Build history of the part. All positions in model axes, mm. Face numbers are marked on the shaded views. Round coordinates to 2 decimals unless told otherwise and drop trailing zeros. Write each loop counter-clockwise with the first axis right and the second up, starting at its lowest first coordinate (ties: lowest second). Pieces come first, ordered by that corner, then holes. Notation, with made-up numbers: M 72.5,38.5 L 118.5,38.5 A25 ccw 118.5,76.5 Z; hole C -20.5,52 d9. An arc over 180 degrees is marked long. Write item = value, one per line. Start each with the question number.
Q1. Band-saw the part on A-A on x = 11.25. Write the cut outline in (y, z), plus the area to 3 significant figures.
Q2. Band-saw the part on C-C on z = -12. Write the cut outline in (x, y), plus the area to 3 significant figures.
Q3. Band-saw the part on B-B on y = 0.9. State how many separate pieces and enclosed holes the cut face has, plus the area to 3 significant figures.
Q4. Drop flat-ended pins along their axis: P1, Ø0.5, axis at x = 11.5, y = 1, coming from the +Z side; P2, Ø5, axis at x = 6.5, z = -112.5, coming from the +Y side; P3, Ø0.8, axis at y = 0.5, z = -6.5, coming from the -X side. Give the stop position or say it passes through.
Q5. Pull direction Z, two halves, no side cores. Call the marked faces 1 and 2: released by +Z, released by -Z, zero draft, split by the parting line, or undercut.
Q6. Probe L1, parallel to Z at x = 16.5, y = 1.1; L2, parallel to Z at x = 8.75, y = 0.7; L3, parallel to Z at x = 6.5, y = 0.6. List the from-to ranges inside material, lowest first.
Q7. Band-saw the part on D-D on z = -114.5. Write the cut outline in (x, y).
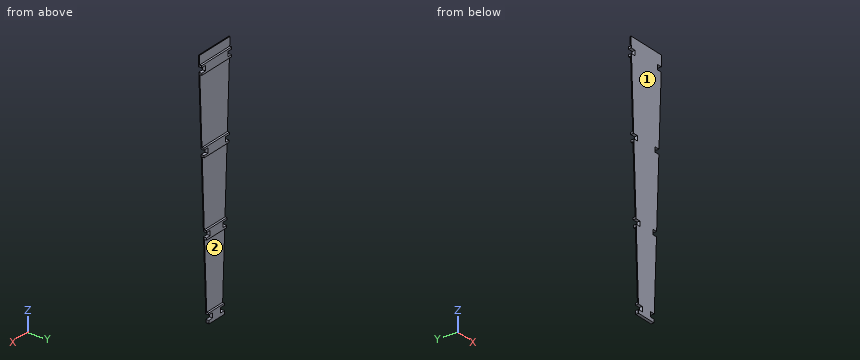
```python
from build123d import *

# Parameters (mm, degrees)
BOSS_EXTRUDE1_DEPTH = 0.5
BOSS_EXTRUDE2_DEPTH = 1


with BuildPart() as part:
    # Sketch2 → Boss-Extrude1 (new body)
    with BuildSketch(Plane(origin=(0, 0, 0), x_dir=(1, 0, 0), z_dir=(0, 1, 0))):
        Polygon((0.216060204, 5.401505112), (0, 0), (20, 0), (19.783939796, 5.401505112), (17.280808425, 5.401505112), (17.280808425, 7.904636482), (19.683814541, 7.904636482), (18.245170319, 43.870742022), (15.742038949, 43.870742022), (15.742038949, 46.373873393), (18.145045064, 46.373873393), (16.706400843, 82.339978933), (14.203269472, 82.339978933), (14.203269472, 84.843110303), (16.606275588, 84.843110303), (15.167631366, 120.809215844), (12.664499996, 120.809215844), (12.664499996, 123.312347214), (15.067506111, 123.312347214), (15, 125), (5, 125), (4.932493889, 123.312347214), (7.335500004, 123.312347214), (7.335500004, 120.809215844), (4.832368634, 120.809215844), (3.393724412, 84.843110303), (5.796730528, 84.843110303), (5.796730528, 82.339978933), (3.293599157, 82.339978933), (1.854954936, 46.373873393), (4.257961051, 46.373873393), (4.257961051, 43.870742022), (1.754829681, 43.870742022), (0.316185459, 7.904636482), (2.719191575, 7.904636482), (2.719191575, 5.401505112), align=None)
    extrude(amount=BOSS_EXTRUDE1_DEPTH)

    # Sketch3 → Boss-Extrude2 (add)
    with BuildSketch(Plane(origin=(0, 0.5, 0), x_dir=(1, 0, 0), z_dir=(0, 1, 0))):
        Polygon((0.216060204, 5.401505112), (0.176060204, 4.401505112), (19.823939796, 4.401505112), (19.783939796, 5.401505112), (17.280808425, 5.401505112), (17.280808425, 7.904636482), (19.683814541, 7.904636482), (19.643814541, 8.904636482), (0.356185459, 8.904636482), (0.316185459, 7.904636482), (2.719191575, 7.904636482), (2.719191575, 5.401505112), align=None)
        Polygon((1.754829681, 43.870742022), (1.716060204, 42.901505112), (18.283939796, 42.901505112), (18.245170319, 43.870742022), (15.742038949, 43.870742022), (15.742038949, 46.373873393), (18.145045064, 46.373873393), (18.103814541, 47.404636482), (1.896185459, 47.404636482), (1.854954936, 46.373873393), (4.257961051, 46.373873393), (4.257961051, 43.870742022), align=None)
        Polygon((3.293599157, 82.339978933), (3.256060204, 81.401505112), (16.743939796, 81.401505112), (16.706400843, 82.339978933), (14.203269472, 82.339978933), (14.203269472, 84.843110303), (16.606275588, 84.843110303), (16.563814541, 85.904636482), (3.436185459, 85.904636482), (3.393724412, 84.843110303), (5.796730528, 84.843110303), (5.796730528, 82.339978933), align=None)
        Polygon((4.832368634, 120.809215844), (4.796060204, 119.901505112), (15.203939796, 119.901505112), (15.167631366, 120.809215844), (12.664499996, 120.809215844), (12.664499996, 123.312347214), (15.067506111, 123.312347214), (15.023814541, 124.404636482), (4.976185459, 124.404636482), (4.932493889, 123.312347214), (7.335500004, 123.312347214), (7.335500004, 120.809215844), align=None)
        Polygon((5, 125), (4.976185459, 124.404636482), (15.023814541, 124.404636482), (15, 125), align=None)
    extrude(amount=BOSS_EXTRUDE2_DEPTH)


solid = part.part
```
Conclusion:
q1.outline = M 0,-125 L 1.5,-125 L 1.5,-119.9 L 0.5,-119.9 L 0.5,-85.9 L 1.5,-85.9 L 1.5,-81.4 L 0.5,-81.4 L 0.5,-47.4 L 1.5,-47.4 L 1.5,-42.9 L 0.5,-42.9 L 0.5,-8.9 L 1.5,-8.9 L 1.5,-4.4 L 0.5,-4.4 L 0.5,0 L 0,0 Z
q1.area = 81.1 mm^2
q2.outline = M 0.48,0 L 19.52,0 L 19.52,0.5 L 0.48,0.5 Z
q2.area = 9.52 mm^2
q3.separate_pieces = 4
q3.enclosed_holes = 0
q3.area = 224 mm^2
q4.P1 = -4.4
q4.P2 = 0.5
q4.P3 = 2.72
q5.face_1 = zero draft
q5.face_2 = undercut
q6.L1 = -85.9 to -84.84, -82.34 to -81.4, -47.4 to -46.37, -43.87 to -42.9, -8.9 to -4.4
q6.L2 = -125 to -119.9, -85.9 to -81.4, -47.4 to -42.9, -8.9 to -4.4
q6.L3 = -125 to -123.31, -120.81 to -119.9, -85.9 to -81.4, -47.4 to -42.9, -8.9 to -4.4
q7.outline = M 4.58,0 L 15.42,0 L 15.42,0.5 L 4.58,0.5 Z
